from build123d import *

# Parameters (mm, degrees)
F0_R      = 10.31875
F1_DEPTH  = 27.7622
F2_T      = -1.2446
F3_R      = 10.0203
F4_DEPTH  = 2.3622
F8_R      = 1.9812
F9_DEPTH  = 12.443506
F10_R     = 1.9812
F11_DEPTH = 12.308541
F13_R     = 1.9812
F14_DEPTH = 12.376495


with BuildPart() as f1:
    # F0 (on Top) → F1 (new body)
    with BuildSketch(Plane.XY):
        Circle(F0_R)
    extrude(amount=F1_DEPTH)

    # F2
    f2_openings = [f1.faces().sort_by_distance(p)[0] for p in [
        (0, 0, 27.7622),
        (0, 0, 0),
    ]]
    offset(amount=F2_T, openings=f2_openings)

    # F3 (on face) → F4 (cut)
    with BuildSketch(Plane(origin=(0, 0, 0), x_dir=(1, 0, 0), z_dir=(0, 0, -1))):
        Circle(F3_R)
    extrude(amount=-F4_DEPTH, mode=Mode.SUBTRACT)

    # F8 (on face) → F9 (cut, through all)
    with BuildSketch(Plane(origin=(0, 0, 0), x_dir=(-0.97237, -0.233445, 0), z_dir=(-0.233445, 0.97237, 0))):
        with Locations((0, 23.79345)):
            Circle(F8_R)
    extrude(amount=-F9_DEPTH, mode=Mode.SUBTRACT)

    # F10 (on face) → F11 (cut, through all)
    with BuildSketch(Plane(origin=(0, 0, 0), x_dir=(-0.976296, -0.21644, 0), z_dir=(-0.21644, 0.976296, 0))):
        with Locations((0, 23.79345)):
            Circle(F10_R)
    extrude(amount=-F11_DEPTH, mode=Mode.SUBTRACT)

    # F13 (on face) → F14 (cut, through all)
    with BuildSketch(Plane(origin=(0, 0, 0), x_dir=(-0.97437, -0.224951, 0), z_dir=(-0.224951, 0.97437, 0))):
        with Locations((0, 23.79345)):
            Circle(F13_R)
    extrude(amount=-F14_DEPTH, mode=Mode.SUBTRACT)


solid = f1.part
Model file for the job. Use its own axes, mm. A direction names the side the tool comes from. Give positions to 0.01 mm unless a question says otherwise; leave off trailing zeros. Order: outer loops, then holes, each group sorted by start corner. A loop starts at its lowest first (then second) coordinate and runs counter-clockwise, first axis right, second up. Notation, with made-up numbers: (52, 55.5) - (86, 55.5) arc R11 cw to (86, 66.5) - close; hole circle Ø9 at (20, 7). An arc over 180 degrees is marked (long way). One line per item, written item: value.
Item 1: Slice it at A-A (y = 0). List the corners of the cut face in (x, z).
Response values:
outline: (-10.32, 0) - (-10.02, 0) - (-10.02, 2.36) - (-9.07, 2.36) - (-9.07, 27.76) - (-10.32, 27.76) - close; (9.07, 2.36) - (10.02, 2.36) - (10.02, 0) - (10.32, 0) - (10.32, 27.76) - (9.07, 27.76) - close
Item 2: Wall check: line 1 (Y direction, x = 0, z = 21); line 2 (X direction, y = 3.75, z = 6.25); line 3 (X direction, y = -3.5, z = 25). Give the ranges that are in metal, low to high.
Response values:
line 1: -10.32 to -9.07, 9.07 to 10.32
line 2: -9.61 to -8.26, 8.26 to 9.61
line 3: -9.71 to -8.37, 8.37 to 9.71
Item 3: Pin check, flat tips, straight feed: pin 1 Ø4 at (x, y) = (-4, 6) entering from -Z; pin 2 Ø10 at (x, y) = (-8, -3.5) entering from +Z; pin 3 Ø6 at (x, z) = (8, 18.5) entering from -Y; pin 4 Ø4 at (x, z) = (-3.5, 11) entering from -Y. Stop position of each tip, or through.
Response values:
pin 1: z = 2.36
pin 2: z = 27.76
pin 3: y = -9.03
pin 4: y = -10.21
Item 4: Slice it at C-C (z = 13.5). List the corners of the cut face in (x, y), then the cut area to 3 significant figures.
Response values:
outline: circle Ø20.64 at (0, 0); hole circle Ø18.15 at (0, 0)
area: 75.8 mm2
Item 5: Slice it at B-B (x = 8.5). List the corners of the cut face in (y, z).
Response values:
outline: (-5.85, 0) - (-5.31, 0) - (-5.31, 2.36) - (-3.18, 2.36) - (-3.18, 27.76) - (-5.85, 27.76) - close; (3.18, 2.36) - (5.31, 2.36) - (5.31, 0) - (5.85, 0) - (5.85, 27.76) - (3.18, 27.76) - close
Item 6: Two-plate mould, pull along Y, no slides. Class faces 1 (the flat face through (-9, -2.3, 2.362)), 2 (the cylindrical face through (-2.237, -10.073, 13.687)), 3 (the cylindrical face through (-2.172, 9.782, 1.165)), 4 (the flat face through (5, -8, 27.762)): released by +Y, released by -Y, zero draft, split by the parting line, or undercut.
Response values:
face 1: undercut
face 2: split by the parting line
face 3: undercut
face 4: zero draft
Item 7: Tool access for faces 5 (the cylindrical face through (-7.2, -5.52, 14.88)), 6 (the cylindrical face through (0.14, -9.78, 23.75)): list every direction of +Z, -Z, +X, -X, +Y, -Y with a clear straight run to the whole face (end or side of a thin tool).
Response values:
face 5: +Z, -Z
face 6: none
